```python
from build123d import *

# Parameters (mm, degrees)
EXTRUDE_1_DEPTH = 5


with BuildPart() as part:
    # 草图1 → 凸台-拉伸1 (new body)
    with BuildSketch(Plane.XY):
        with BuildLine():
            Line((95.989328864, 7.5), (14, 7.5))
            ThreePointArc((14, 7.5), (11, 2.303847577), (5, 2.303847577))
            Line((5, 2.303847577), (5, 0))
            Line((5, 0), (105, 0))
            Line((105, 0), (105, 2.291529254))
            ThreePointArc((105, 2.291529254), (98.991997831, 2.296146576), (95.989328864, 7.5))
        make_face()
        with BuildLine():
            ThreePointArc((5, 2.303847577), (2.803847577, 4.5), (2, 7.5))
            Line((2, 7.5), (0, 7.5))
            Line((0, 7.5), (0, 5))
            ThreePointArc((0, 5), (1.464466094, 1.464466094), (5, 0))
            Line((5, 0), (5, 2.303847577))
        make_face()
        with BuildLine():
            Line((5, 12.696152423), (5, 15))
            ThreePointArc((5, 15), (1.464466094, 13.535533906), (0, 10))
            Line((0, 10), (0, 7.5))
            Line((0, 7.5), (2, 7.5))
            ThreePointArc((2, 7.5), (2.803847577, 10.5), (5, 12.696152423))
        make_face()
        with BuildLine():
            Line((105, 15), (5, 15))
            Line((5, 15), (5, 12.696152423))
            ThreePointArc((5, 12.696152423), (11, 12.696152423), (14, 7.5))
            Line((14, 7.5), (95.989328864, 7.5))
            ThreePointArc((95.989328864, 7.5), (98.991997831, 12.703853424), (105, 12.708470746))
            Line((105, 12.708470746), (105, 15))
        make_face()
        with BuildLine():
            ThreePointArc((110, 10), (108.535533906, 13.535533906), (105, 15))
            Line((105, 15), (105, 12.708470746))
            ThreePointArc((105, 12.708470746), (107.203853424, 10.508002169), (108.010671136, 7.5))
            Line((108.010671136, 7.5), (110, 7.5))
            Line((110, 7.5), (110, 10))
        make_face()
        with BuildLine():
            Line((110, 7.5), (108.010671136, 7.5))
            ThreePointArc((108.010671136, 7.5), (107.203853424, 4.491997831), (105, 2.291529254))
            Line((105, 2.291529254), (105, 0))
            ThreePointArc((105, 0), (108.535533906, 1.464466094), (110, 5))
            Line((110, 5), (110, 7.5))
        make_face()
    extrude(amount=EXTRUDE_1_DEPTH)


solid = part.part
```
Work out the finished part from the listing and answer in its coordinate system (mm). Round coordinates to 2 decimals unless told otherwise and drop trailing zeros. Write each loop counter-clockwise with the first axis right and the second up, starting at its lowest first coordinate (ties: lowest second). Pieces come first, ordered by that corner, then holes. Notation, with made-up numbers: (83.5, 51.5) -> (129.5, 51.5) arc R21 cw to (129.5, 83.5) -> close; hole circle Ø11 at (56.25, 29). An arc over 180 degrees is marked (long way). Write each question's results on one line, items separated by ' | '.
1) The part is cut by section D-D (y = 11.75). Write down the section's boundary in (x, z).
Findings:
outline: (0.32, 0) -> (3.76, 0) -> (3.76, 5) -> (0.32, 5) -> close; (12.24, 0) -> (97.75, 0) -> (97.75, 5) -> (12.24, 5) -> close; (106.25, 0) -> (109.68, 0) -> (109.68, 5) -> (106.25, 5) -> close
2) Consider line 1 along X through (y, z) = (7, 4.3); line 2 along X through (y, z) = (2.5, 1.9); line 3 along Y through (x, z) = (101.5, 4.35). Determine where each line is inside the solid, lowest interval first. Write a range as [from, to].
Findings:
line 1: x = [0, 2.02], [13.98, 96.01], [107.99, 110] | line 2: x = [0.67, 4.68], [11.32, 98.66], [105.34, 109.33] | line 3: y = [0, 1.51], [13.49, 15]
3) The part is cut by section A-A (x = 12). Write down the section's boundary in (y, z).
Findings:
outline: (0, 0) -> (3.03, 0) -> (3.03, 5) -> (0, 5) -> close; (11.97, 0) -> (15, 0) -> (15, 5) -> (11.97, 5) -> close
4) The part is cut by section B-B (z = 0.8). Write down the section's boundary in (x, y), and give its area (3 significant figures).
Findings:
outline: (0, 5) arc R5 ccw to (5, 0) -> (105, 0) arc R5 ccw to (110, 5) -> (110, 10) arc R5 ccw to (105, 15) -> (5, 15) arc R5 ccw to (0, 10) -> close; hole circle Ø12 at (8, 7.5); hole circle Ø12.02 at (102, 7.5) | area: 1,400 mm²
5) The part is cut by section C-C (y = 6.5). Write down the section's boundary in (x, z).
Findings:
outline: (0, 0) -> (2.08, 0) -> (2.08, 5) -> (0, 5) -> close; (13.92, 0) -> (96.07, 0) -> (96.07, 5) -> (13.92, 5) -> close; (107.93, 0) -> (110, 0) -> (110, 5) -> (107.93, 5) -> close
